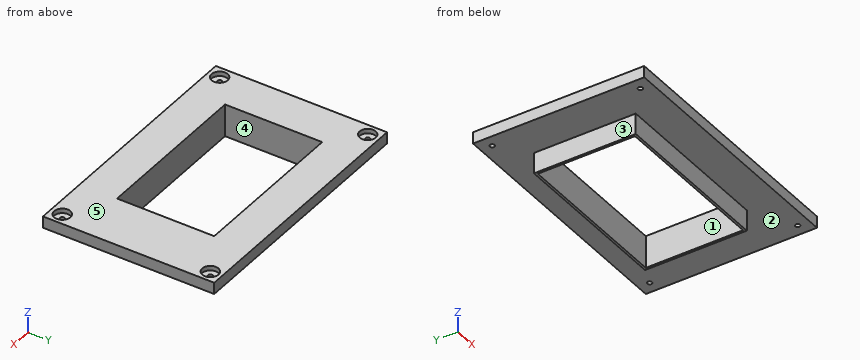
```python
from build123d import *

# Parameters (mm, degrees)
SKETCH_W        = 112
SKETCH_H        = 74
SKETCH_R        = 1
PAD_DEPTH       = 5
SKETCH001_R     = 3.5
POCKET_DEPTH    = 2
SKETCH002_W     = 70
SKETCH002_H     = 42
POCKET001_DEPTH = 5
SKETCH003_W     = 72
SKETCH003_H     = 44
SKETCH003_W_2   = 70
SKETCH003_H_2   = 42
PAD001_DEPTH    = 9


with BuildPart() as part:
    # Sketch → Pad (new body)
    with BuildSketch(Plane.XY):
        with Locations((56, 37)):
            Rectangle(SKETCH_W, SKETCH_H)
        with Locations((5, 69)):
            Circle(SKETCH_R, mode=Mode.SUBTRACT)
        with Locations((5, 5)):
            Circle(SKETCH_R, mode=Mode.SUBTRACT)
        with Locations((107, 69)):
            Circle(SKETCH_R, mode=Mode.SUBTRACT)
        with Locations((107, 5)):
            Circle(SKETCH_R, mode=Mode.SUBTRACT)
    extrude(amount=PAD_DEPTH)

    # Sketch001 → Pocket (cut)
    with BuildSketch(Plane.XY.offset(5)):
        with Locations((5, 5)):
            Circle(SKETCH001_R)
        with Locations((5, 69)):
            Circle(SKETCH001_R)
        with Locations((107, 69)):
            Circle(SKETCH001_R)
        with Locations((107, 5)):
            Circle(SKETCH001_R)
    extrude(amount=-POCKET_DEPTH, mode=Mode.SUBTRACT)

    # Sketch002 → Pocket001 (cut)
    with BuildSketch(Plane.XY.offset(5)):
        with Locations((53, 37)):
            Rectangle(SKETCH002_W, SKETCH002_H)
    extrude(amount=-POCKET001_DEPTH, mode=Mode.SUBTRACT)

    # Sketch003 → Pad001 (new body)
    with BuildSketch(Plane(origin=(0, 0, 0), x_dir=(1, 0, 0), z_dir=(0, 0, -1))):
        with Locations((53, -37)):
            Rectangle(SKETCH003_W, SKETCH003_H)
        with Locations((53, -37)):
            Rectangle(SKETCH003_W_2, SKETCH003_H_2, mode=Mode.SUBTRACT)
    extrude(amount=PAD001_DEPTH)


solid = part.part
```
Design review of the part built by this model. Coordinates are the model's own, in mm. Face numbers are marked on the shaded views. A direction names the side the tool comes from. Coordinates: 2 decimals unless noted, no trailing zeros. Write each loop counter-clockwise with the first axis right and the second up, starting at its lowest first coordinate (ties: lowest second). Pieces come first, ordered by that corner, then holes.
1) To check wall thickness, follow L1, parallel to X at y = 5, z = 1.75; L2, parallel to Y at x = 107, z = 1.65; L3, parallel to Y at x = 5, z = 4.1. State the ranges of each line that lie inside material, in increasing order.
2) Add section B-B (y = 30.5). Write out the cut boundary in (x, z).
3) Add section C-C (x = 99.5). Write out the cut boundary in (y, z).
4) Add section A-A (z = -4). Write out the cut boundary in (x, y), plus the area to 3 significant figures.
5) Mouldability with a two-part tool opening along X and no side actions: class the marked faces 1, 2 and 3 as +X half, -X half, draft (parallel to the pull), parting line (faces both ways), or undercut.
6) Insertion check: pin 1 (5 mm diameter, centred on y = 23, z = -3, fed in from -X); pin 2 (10 mm diameter, centred on x = 75.5, y = 18.5, fed in from +Z); pin 3 (6.5 mm diameter, centred on x = 107, y = 5, fed in from -Z); pin 4 (4.5 mm diameter, centred on x = 47.5, z = -5.5, fed in from -Y). Each pin has a flat end and moves straight along its axis. Give the tip position at first contact, or say it passes through.
7) Machinability: for the marked faces 4 and 5, which of the approach directions +Z, -Z, +X, -X, +Y, -Y give a long, thin tool a straight path to every point of the face, cutting with its end or side? Answer none if there is none.
Check result:
1. L1: x = 0 to 4, 6 to 106, 108 to 112
1. L2: y = 0 to 4, 6 to 68, 70 to 74
1. L3: y = 0 to 1.5, 8.5 to 65.5, 72.5 to 74
2. outline: (0, 0) - (17, 0) - (17, -9) - (18, -9) - (18, 5) - (0, 5) - close; (88, -9) - (89, -9) - (89, 0) - (112, 0) - (112, 5) - (88, 5) - close
3. outline: (0, 0) - (74, 0) - (74, 5) - (0, 5) - close
4. outline: (17, 15) - (89, 15) - (89, 59) - (17, 59) - close; hole (18, 16) - (88, 16) - (88, 58) - (18, 58) - close
4. area: 228 mm2
5. face 1: undercut
5. face 2: draft
5. face 3: -X half
6. pin 1: stops at x = 17
6. pin 2: stops at z = 5
6. pin 3: stops at z = 0
6. pin 4: stops at y = 15
7. face 4: +Z, -Z
7. face 5: +Z, +X, -X, +Y, -Y
